```python
from build123d import *

# Parameters (mm, degrees)
SKETCH2_W           = 73
SKETCH2_H           = 28
BOSS_EXTRUDE1_DEPTH = 5
CUT_EXTRUDE2_START  = 36.5
SKETCH3_R           = 2
CUT_EXTRUDE2_DEPTH  = 5
BOSS_EXTRUDE2_START = -36.5
SKETCH3_2_R         = 2
BOSS_EXTRUDE2_DEPTH = 10
BOSS_EXTRUDE3_START = -36.5
SKETCH3_3_R         = 2
BOSS_EXTRUDE3_DEPTH = 5


with BuildPart() as part:
    # Sketch2 → Boss-Extrude1 (new, symmetric)
    with BuildSketch(Plane(origin=(0, 0, 0), x_dir=(1, 0, 0), z_dir=(0, 1, 0))):
        Rectangle(SKETCH2_W, SKETCH2_H)
    extrude(amount=BOSS_EXTRUDE1_DEPTH, both=True)

    # Sketch3 → Cut-Extrude2 (cut)
    with BuildSketch(Plane(origin=(0, 0, 0), x_dir=(0, 0, -1), z_dir=(1, 0, 0)).offset(CUT_EXTRUDE2_START)):
        with Locations(Location((0, 0, 0), (0, 0, 180))):
            Circle(SKETCH3_R)
        with Locations(Location((11.75, 0, 0), (0, 0, 180))):
            Circle(SKETCH3_R)
        with Locations(Location((-11.75, 0, 0), (0, 0, 180))):
            Circle(SKETCH3_R)
    extrude(amount=-CUT_EXTRUDE2_DEPTH, mode=Mode.SUBTRACT)

    # Sketch3<2> → Boss-Extrude2 (add, symmetric)
    with BuildSketch(Plane(origin=(0, 0, 0), x_dir=(0, 0, -1), z_dir=(1, 0, 0)).offset(BOSS_EXTRUDE2_START)):
        with Locations(Location((11.75, 0, 0), (0, 0, 180))):
            Circle(SKETCH3_2_R)
        with Locations(Location((-11.75, 0, 0), (0, 0, 180))):
            Circle(SKETCH3_2_R)
    extrude(amount=BOSS_EXTRUDE2_DEPTH, both=True)

    # Sketch3<3> → Boss-Extrude3 (add, symmetric)
    with BuildSketch(Plane(origin=(0, 0, 0), x_dir=(0, 0, -1), z_dir=(1, 0, 0)).offset(BOSS_EXTRUDE3_START)):
        with Locations(Location((0, 0, 0), (0, 0, 180))):
            Circle(SKETCH3_3_R)
    extrude(amount=BOSS_EXTRUDE3_DEPTH, both=True)


solid = part.part
```
Check sheet for the modelled part. Datum: model origin and axes. Units: mm. A direction names the side the tool comes from. Round coordinates to 2 decimals unless told otherwise and drop trailing zeros. Order: outer loops, then holes, each group sorted by start corner. A loop starts at its lowest first (then second) coordinate and runs counter-clockwise, first axis right, second up. Notation, with made-up numbers: M 45.5,-16 L 97.5,-16 A27 cw 97.5,4 Z; hole C -5,-34 d9. An arc over 180 degrees is marked long. Answer in a Markdown table with one row per item.
(1) Section check A-A on z = -11.75. Record the boundary of the cut face in (x, y).
Findings:
| item | result |
|---|---|
| outline | M -46.5,-2 L -36.5,-2 L -36.5,-5 L 36.5,-5 L 36.5,-2 L 31.5,-2 L 31.5,2 L 36.5,2 L 36.5,5 L -36.5,5 L -36.5,2 L -46.5,2 Z |
(2) Gauge pin test, flat ends, axial feed: pin 1 (3 mm diameter, centred on y = -0.5, z = -2, fed in from -X); pin 2 (1 mm diameter, centred on y = 0, z = -10.5, fed in from +X). Record the tip position at first contact, or that the pin passes through.
Findings:
| item | result |
|---|---|
| pin 1 | stops at x = -41.5 |
| pin 2 | stops at x = 31.5 |
(3) Set-up check for faces 1 (the flat face through (-46.5, 0, 12)), 2 (the cylindrical face through (34.035, 1.217, 10.163)), 3 (the cylindrical face through (-39, 2, 0)), 4 (the flat face through (-41.5, 0, 0)): record each of +Z, -Z, +X, -X, +Y, -Y from which the full face is reachable in a straight line by a thin tool's end or side.
Findings:
| item | result |
|---|---|
| face 1 | +Z, -Z, -X, +Y, -Y |
| face 2 | +X |
| face 3 | -X |
| face 4 | -X, +Y, -Y |
(4) Material ranges on line 1 along Y through (x, z) = (32.6, -11.75); line 2 along X through (y, z) = (0.75, 4); line 3 along X through (y, z) = (-0.5, -10.5), recorded low to high. Write a range as from..to.
Findings:
| item | result |
|---|---|
| line 1 | y = -5..-2, 2..5 |
| line 2 | x = -36.5..36.5 |
| line 3 | x = -46.5..31.5 |
(5) Draft check along Y on faces 5 (the cylindrical face through (34.035, 1.217, -13.337)), 6 (the cylindrical face through (-41.43, 1.217, -13.337)), 7 (the flat face through (-46.5, 0, -12)), 8 (the flat face through (-1, 5, 0)). Enter one of: +Y half, -Y half, draft (parallel to the pull), parting line (faces both ways), or undercut.
Findings:
| item | result |
|---|---|
| face 5 | undercut |
| face 6 | parting line |
| face 7 | draft |
| face 8 | +Y half |
(6) Section check B-B on x = -40. Record the boundary of the cut face in (y, z).
Findings:
| item | result |
|---|---|
| outline | C 0,-11.75 d4; C 0,0 d4; C 0,11.75 d4 |
(7) Section check D-D on z = 0. Record the boundary of the cut face in (x, y).
Findings:
| item | result |
|---|---|
| outline | M -41.5,-2 L -36.5,-2 L -36.5,-5 L 36.5,-5 L 36.5,-2 L 31.5,-2 L 31.5,2 L 36.5,2 L 36.5,5 L -36.5,5 L -36.5,2 L -41.5,2 Z |
(8) Section check C-C on y = 0. Record the boundary of the cut face in (x, z).
Findings:
| item | result |
|---|---|
| outline | M -46.5,-13.75 L -36.5,-13.75 L -36.5,-14 L 36.5,-14 L 36.5,-13.75 L 31.5,-13.75 L 31.5,-9.75 L 36.5,-9.75 L 36.5,-2 L 31.5,-2 L 31.5,2 L 36.5,2 L 36.5,9.75 L 31.5,9.75 L 31.5,13.75 L 36.5,13.75 L 36.5,14 L -36.5,14 L -36.5,13.75 L -46.5,13.75 L -46.5,9.75 L -36.5,9.75 L -36.5,2 L -41.5,2 L -41.5,-2 L -36.5,-2 L -36.5,-9.75 L -46.5,-9.75 Z |
